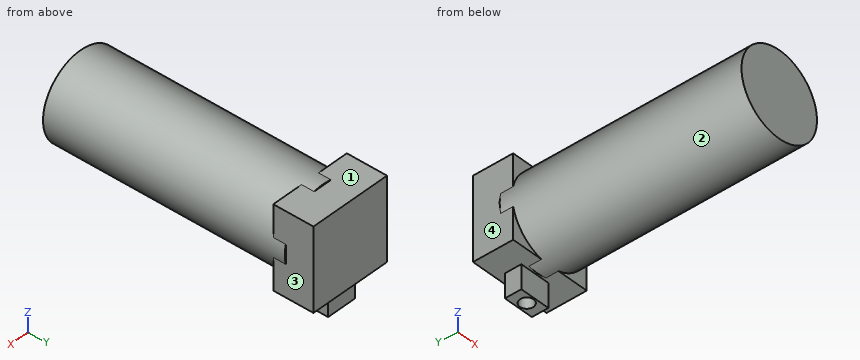
from build123d import *

# Parameters (mm, degrees)
SKETCH_W     = 38
SKETCH_H     = 38
PAD_DEPTH    = 18.6
SKETCH001_W  = 13.97
SKETCH001_H  = 12
PAD001_DEPTH = 7.62
SKETCH002_R  = 19.5
PAD002_DEPTH = 112
SKETCH003_R  = 3.175
POCKET_DEPTH = 20


with BuildPart() as part:
    # Sketch → Pad (new body)
    with BuildSketch(Plane.XZ):
        Rectangle(SKETCH_W, SKETCH_H)
    extrude(amount=PAD_DEPTH)

    # Sketch001 → Pad001 (join)
    with BuildSketch(Plane.XZ.offset(3.98)):
        with Locations((0, -24)):
            Rectangle(SKETCH001_W, SKETCH001_H)
    extrude(amount=PAD001_DEPTH)

    # Sketch002 → Pad002 (join)
    with BuildSketch(Plane.XZ.offset(12.8)):
        Circle(SKETCH002_R)
    extrude(amount=PAD002_DEPTH)

    # Sketch003 → Pocket (cut)
    with BuildSketch(Plane.XY.offset(-20)):
        with Locations((0, -7.85)):
            Circle(SKETCH003_R)
    extrude(amount=-POCKET_DEPTH, mode=Mode.SUBTRACT)


solid = part.part
Read the model definition and answer for the solid it produces. Units are mm, in the model's axes. Face numbers are marked on the shaded views. A direction names the side the tool comes from. Coordinates: 2 decimals unless noted, no trailing zeros. Loops run counter-clockwise (first coordinate to the right, second up) from the corner with the lowest first, then second, coordinate; pieces in that order, holes last. Notation, with made-up numbers: (85.25, 33) -> (100.25, 33) arc R7 cw to (100.25, 39) -> close; hole circle Ø6 at (36.5, 86.5). An arc over 180 degrees is marked (long way). Answer in a Markdown table with one row per item.
Item 1: Straight lines are drawn through the part: line 1 along Y through (x, z) = (0, -25) (3 decimals); line 2 along X through (y, z) = (-116.5, 1); line 3 along Z through (x, y) = (12, -10). For each, find the intervals that lie inside material, in ascending order. Write a range as [from, to].
Returned:
| item | result |
|---|---|
| line 1 | y = [-11.6, -11.025], [-4.675, -3.98] |
| line 2 | x = [-19.47, 19.47] |
| line 3 | z = [-19, 19] |
Item 2: For the marked faces 1, 2, 3 and 4, determine the directions among +Z, -Z, +X, -X, +Y, -Y from which every point of the face is accessible in a straight line to the end or side of a thin tool.
Returned:
| item | result |
|---|---|
| face 1 | +Z, +Y |
| face 2 | -Y |
| face 3 | +X, +Y |
| face 4 | -X, +Y |
Item 3: A cutting plane is placed at D-D on z = -16. Determine the outline of the cut face in (x, y).
Returned:
| item | result |
|---|---|
| outline | (-19, -18.6) -> (-11.15, -18.6) -> (-11.15, -124.8) -> (11.15, -124.8) -> (11.15, -18.6) -> (19, -18.6) -> (19, 0) -> (-19, 0) -> close |
Item 4: A cutting plane is placed at B-B on y = -7.85. Determine the outline of the cut face in (x, z) (3 decimals), plus the area to 3 significant figures.
Returned:
| item | result |
|---|---|
| outline | (-19, -19) -> (-6.985, -19) -> (-6.985, -30) -> (-3.175, -30) -> (-3.175, -20) -> (3.175, -20) -> (3.175, -30) -> (6.985, -30) -> (6.985, -19) -> (19, -19) -> (19, 19) -> (-19, 19) -> close |
| area | 1,530 mm^2 |
Item 5: A cutting plane is placed at C-C on x = 0. Determine the outline of the cut face in (y, z) (3 decimals), plus the area to 3 significant figures.
Returned:
| item | result |
|---|---|
| outline | (-124.8, -19.5) -> (-12.8, -19.5) -> (-12.8, -19) -> (-11.6, -19) -> (-11.6, -30) -> (-11.025, -30) -> (-11.025, -20) -> (-4.675, -20) -> (-4.675, -30) -> (-3.98, -30) -> (-3.98, -19) -> (0, -19) -> (0, 19) -> (-12.8, 19) -> (-12.8, 19.5) -> (-124.8, 19.5) -> close |
| area | 4,870 mm^2 |
Item 6: Each of these flat-tipped pins is pushed along its axis until it touches: P1, Ø10, axis at x = 6.5, y = -95, coming from the +Z side; P2, Ø5.5, axis at x = -1.5, z = -26, coming from the +Y side; P3, Ø4, axis at y = -9.5, z = -23, coming from the +X side (3 decimals). Where does it stop, or does it pass through?
Returned:
| item | result |
|---|---|
| P1 | stops at z = 19.44 |
| P2 | stops at y = -3.98 |
| P3 | stops at x = 6.985 |
Item 7: A cutting plane is placed at A-A on z = -23. Determine the outline of the cut face in (x, y) (3 decimals), plus the area to 3 significant figures.
Returned:
| item | result |
|---|---|
| outline | (-6.985, -11.6) -> (6.985, -11.6) -> (6.985, -3.98) -> (-6.985, -3.98) -> close; hole circle Ø6.35 at (0, -7.85) |
| area | 74.8 mm^2 |
